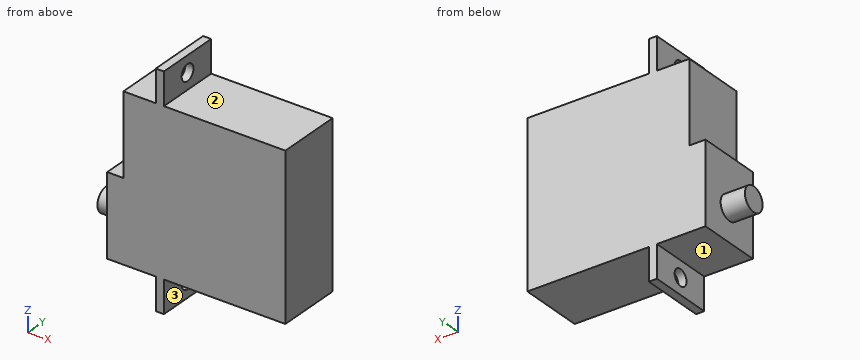
from build123d import *

# Parameters (mm, degrees)
SKETCH1_W           = 20
SKETCH1_H           = 20
BOSS_EXTRUDE1_DEPTH = 8
SKETCH2_W           = 1
SKETCH2_H           = 8
BOSS_EXTRUDE2_DEPTH = 4
SKETCH3_W           = 1
SKETCH3_H           = 8
BOSS_EXTRUDE3_DEPTH = 4
SKETCH4_R           = 1
CUT_EXTRUDE1_DEPTH  = 4
SKETCH5_W           = 10
SKETCH5_H           = 8
BOSS_EXTRUDE4_DEPTH = 2
SKETCH6_R           = 1.5
BOSS_EXTRUDE5_DEPTH = 3


with BuildPart() as part:
    # Sketch1 → Boss-Extrude1 (new body)
    with BuildSketch(Plane(origin=(0, 0, 0), x_dir=(1, 0, 0), z_dir=(0, 1, 0))):
        with Locations((10, -10)):
            Rectangle(SKETCH1_W, SKETCH1_H)
    extrude(amount=BOSS_EXTRUDE1_DEPTH)

    # Sketch2 → Boss-Extrude2 (add)
    with BuildSketch(Plane(origin=(0, 0, 0), x_dir=(-1, 0, 0), z_dir=(0, 0, -1))):
        with Locations((-4.5, 4)):
            Rectangle(SKETCH2_W, SKETCH2_H)
    extrude(amount=BOSS_EXTRUDE2_DEPTH)

    # Sketch3 → Boss-Extrude3 (add)
    with BuildSketch(Plane.XY.offset(20)):
        with Locations((4.5, 4)):
            Rectangle(SKETCH3_W, SKETCH3_H)
    extrude(amount=BOSS_EXTRUDE3_DEPTH)

    # Sketch4 → Cut-Extrude1 (cut)
    with BuildSketch(Plane.ZY.offset(-4)):
        with Locations(Location((-2, 4, 0), (0, 0, 270))):
            Circle(SKETCH4_R)
        with Locations(Location((22, 4, 0), (0, 0, 270))):
            Circle(SKETCH4_R)
    extrude(amount=-CUT_EXTRUDE1_DEPTH, mode=Mode.SUBTRACT)

    # Sketch5 → Boss-Extrude4 (add)
    with BuildSketch(Plane.ZY):
        with Locations((5, 4)):
            Rectangle(SKETCH5_W, SKETCH5_H)
    extrude(amount=BOSS_EXTRUDE4_DEPTH)

    # Sketch6 → Boss-Extrude5 (add)
    with BuildSketch(Plane.ZY.offset(2)):
        with Locations((4, 3.944627207)):
            Circle(SKETCH6_R)
    extrude(amount=BOSS_EXTRUDE5_DEPTH)


solid = part.part
The model under review builds one solid part; all positions refer to its coordinate system, in mm. Face numbers are marked on the shaded views. A direction names the side the tool comes from. Round coordinates to 2 decimals unless told otherwise and drop trailing zeros. Loops run counter-clockwise (first coordinate to the right, second up) from the corner with the lowest first, then second, coordinate; pieces in that order, holes last. Notation, with made-up numbers: (22.25, 47) -> (68.25, 47) arc R7 cw to (68.25, 55) -> close; hole circle Ø5 at (-31, -13). An arc over 180 degrees is marked (long way). Write item = value, one per line. Start each with the question number.
Item 1: For the marked faces 1, 2 and 3, list the 3-axis set-ups (+Z, -Z, +X, -X, +Y, -Y) from which the entire face can be reached by the end or side of a thin tool; tool diameter is ignored.
Item 2: Insertion check: pin 1 (1.8 mm diameter, centred on y = 4, z = 22, fed in from +X); pin 2 (2 mm diameter, centred on x = 2.5, y = 4, fed in from +Z); pin 3 (3 mm diameter, centred on y = 2.5, z = -3, fed in from +X); pin 4 (2 mm diameter, centred on y = 2.5, z = 19.5, fed in from -X). Each pin has a flat end and moves straight along its axis. Give the tip position at first contact, or say it passes through.
Item 3: Take a section at B-B on y = 3.5. Give the boundary of the cut face in (x, z).
Item 4: Take a section at A-A on z = -2. Give the boundary of the cut face in (x, y), plus the area to 3 significant figures.
Item 5: Take a section at C-C on z = 4. Give the boundary of the cut face in (x, y), plus the area to 3 significant figures.
Item 6: Take a section at D-D on y = 1.75. Give the boundary of the cut face in (x, z).
Item 7: To check wall thickness, follow L1, parallel to Z at x = 4.6, y = 4; L2, parallel to X at y = 1.25, z = 11.25. State the ranges of each line that lie inside material, in increasing order.
Result:
q1.face_1 = -Z, -X, +Y, -Y
q1.face_2 = +Z, +X, +Y, -Y
q1.face_3 = -Z, +X, +Y, -Y
q2.pin_1 = through
q2.pin_2 = 20
q2.pin_3 = 5
q2.pin_4 = 0
q3.outline = (-5, 2.57) -> (-2, 2.57) -> (-2, 0) -> (4, 0) -> (4, -1.13) -> (5, -1.13) -> (5, 0) -> (20, 0) -> (20, 20) -> (5, 20) -> (5, 21.13) -> (4, 21.13) -> (4, 20) -> (0, 20) -> (0, 10) -> (-2, 10) -> (-2, 5.43) -> (-5, 5.43) -> close; (4, -4) -> (5, -4) -> (5, -2.87) -> (4, -2.87) -> close; (4, 22.87) -> (5, 22.87) -> (5, 24) -> (4, 24) -> close
q4.outline = (4, 0) -> (5, 0) -> (5, 3) -> (4, 3) -> close; (4, 5) -> (5, 5) -> (5, 8) -> (4, 8) -> close
q4.area = 6.00 mm²
q5.outline = (-5, 2.44) -> (-2, 2.44) -> (-2, 0) -> (20, 0) -> (20, 8) -> (-2, 8) -> (-2, 5.44) -> (-5, 5.44) -> close
q5.area = 185 mm²
q6.outline = (-2, 0) -> (4, 0) -> (4, -4) -> (5, -4) -> (5, 0) -> (20, 0) -> (20, 20) -> (5, 20) -> (5, 24) -> (4, 24) -> (4, 20) -> (0, 20) -> (0, 10) -> (-2, 10) -> close
q7.L1 = -4 to -3, -1 to 21, 23 to 24
q7.L2 = 0 to 20
